from build123d import *

# Parameters (mm, degrees)
BOX013_W     = 32
BOX013_H     = 56
BOX013_DEPTH = 4
BOX002_W     = 170
BOX002_H     = 70
BOX002_DEPTH = 5


with BuildPart() as soporte_motor:
    # Box013 → Box013 (new body)
    with BuildSketch(Plane(origin=(0, -28, 5), x_dir=(1, 0, 0), z_dir=(0, 0, 1))):
        with Locations((16, 28)):
            Rectangle(BOX013_W, BOX013_H)
    extrude(amount=BOX013_DEPTH)


with BuildPart() as obj1:
    # Box002 → Box002 (new body)
    with BuildSketch(Plane(origin=(0, -35, 0), x_dir=(1, 0, 0), z_dir=(0, 0, 1))):
        with Locations((85, 35)):
            Rectangle(BOX002_W, BOX002_H)
    extrude(amount=BOX002_DEPTH)


with BuildPart() as base:
    # Link011 base: copy of soporte motor
    add(soporte_motor.part)


with BuildPart() as base_1:
    # Link011 placement: moved
    add(base.part.moved(Location((138, 0, 0))))

    # Fusion008: union soporte motor, obj1
    add(soporte_motor.part)
    add(obj1.part)


solid = base_1.part
Design review of the part built by this model. Coordinates are the model's own, in mm. A direction names the side the tool comes from. Round coordinates to 2 decimals unless told otherwise and drop trailing zeros. Loops run counter-clockwise (first coordinate to the right, second up) from the corner with the lowest first, then second, coordinate; pieces in that order, holes last. Notation, with made-up numbers: M 70,-27 L 91,-27 A30 ccw 91,4 Z; hole C 66,22.5 d1. An arc over 180 degrees is marked long. Answer as a JSON object with one key per item and string values.
Item 1: The part is to be moulded in two halves that separate along X. For faces 4 (the flat face through (84, 35, 2)), 5 (the flat face through (0, 0, 4)), 6 (the flat face through (32, 0, 7)), say which applies: pulls with the +X half, pulls with the -X half, needs draft (parallel to the pull), parting line crosses it, or undercut.
Answer sheet:
{"face 4": "needs draft", "face 5": "pulls with the -X half", "face 6": "undercut"}
Item 2: Wall thickness on L1, parallel to X at y = 27, z = 7.5; L2, parallel to Z at x = 58.5, y = -32: over which ranges is each line inside the solid? List them lowest first. Write a range as from..to.
Answer sheet:
{"L1": "x = 0..32, 138..170", "L2": "z = 0..5"}
Item 3: Clearance check with flat-ended pins moving along their axes: P1, Ø1.2, axis at x = 147, z = 7, coming from the +Y side; P2, Ø1, axis at x = 41.5, y = -17, coming from the +Z side; P3, Ø1.2, axis at x = 11, z = 8, coming from the -Y side. State where each tip first meets the part, or that it passes through.
Answer sheet:
{"P1": "stops at y = 28", "P2": "stops at z = 5", "P3": "stops at y = -28"}
Item 4: We need section B-B on y = -22. Give the boundary of the cut face in (x, z), and give its area (3 significant figures).
Answer sheet:
{"outline": "M 0,0 L 170,0 L 170,9 L 138,9 L 138,5 L 32,5 L 32,9 L 0,9 Z", "area": "1,110 mm^2"}
Item 5: Machinability: for faces 1 (the flat face through (16, 28, 7)), 2 (the flat face through (16, -28, 7)), 3 (the flat face through (138, 0, 7)), which of the approach directions +Z, -Z, +X, -X, +Y, -Y give a long, thin tool a straight path to every point of the face, cutting with its end or side? Answer none if there is none.
Answer sheet:
{"face 1": "+Z, +X, -X, +Y", "face 2": "+Z, +X, -X, -Y", "face 3": "+Z, +Y, -Y"}
Item 6: We need section A-A on x = 158. Give the boundary of the cut face in (y, z), and give its area (3 significant figures).
Answer sheet:
{"outline": "M -35,0 L 35,0 L 35,5 L 28,5 L 28,9 L -28,9 L -28,5 L -35,5 Z", "area": "574 mm^2"}
Item 7: We need section C-C on x = 52.5. Give the boundary of the cut face in (y, z).
Answer sheet:
{"outline": "M -35,0 L 35,0 L 35,5 L -35,5 Z"}
